from build123d import *

# Parameters (mm, degrees)
SKETCH042_R              = 1.9
PAD007_DEPTH             = 1.9
POCKET024_DEPTH          = 1.2
SKETCH044_R              = 1
PAD008_DEPTH             = 12
FILLET005_R              = 0.2
BODY008_PLACEMENT_ANGLE  = 90
CLONE004_PLACEMENT_ANGLE = 90


with BuildPart() as part:
    # Sketch042 → Pad007 (new body)
    with BuildSketch(Plane.XY):
        Circle(SKETCH042_R)
    extrude(amount=PAD007_DEPTH)

    # Sketch043 (on Face3 of Pad007) → Pocket024 (cut)
    with BuildSketch(Plane.XY.offset(1.9)):
        Polygon((0.866025, 0), (0.433013, 0.75), (-0.433013, 0.75), (-0.866025, 0), (-0.433013, -0.75), (0.433013, -0.75), align=None)
    extrude(amount=-POCKET024_DEPTH, mode=Mode.SUBTRACT)

    # Sketch044 → Pad008 (join)
    with BuildSketch(Plane.XY):
        Circle(SKETCH044_R)
    extrude(amount=-PAD008_DEPTH)

    # Fillet005
    fillet005_edges = [part.edges().sort_by_distance(p)[0] for p in [
        (-1.9, 0, 1.9),
        (-0.649519, 0.375, 1.9),
        (-0.649519, -0.375, 1.9),
        (0, -0.75, 1.9),
        (0.649519, -0.375, 1.9),
        (0.649519, 0.375, 1.9),
        (0, 0.75, 1.9),
    ]]
    fillet(fillet005_edges, radius=FILLET005_R)


with BuildPart() as part_1:
    # Body008 placement: moved
    add(part.part.moved(Location((40, -5, 15))).rotate(Axis((40, -5, 15), (1, 0, 0)), BODY008_PLACEMENT_ANGLE))


with BuildPart() as part_2:
    # Clone004 placement: moved
    add(part_1.part.moved(Location((-40, -15, -5))).rotate(Axis((-40, -15, -5), (-1, 0, 0)), CLONE004_PLACEMENT_ANGLE))


with BuildPart() as part_3:
    # Body011 placement: moved
    add(part_2.part.moved(Location((67, -5, 21))))


solid = part_3.part
The listing builds one solid part. Answer for the finished solid, in the listing's coordinates (mm). A direction names the side the tool comes from. Coordinates: 2 decimals unless noted, no trailing zeros. Loops run counter-clockwise (first coordinate to the right, second up) from the corner with the lowest first, then second, coordinate; pieces in that order, holes last. Notation, with made-up numbers: (26.5, 36.25) -> (35.5, 36.25) arc R7 ccw to (35.5, 48.25) -> close; hole circle Ø2 at (14, 86.5). An arc over 180 degrees is marked (long way). Answer in a Markdown table with one row per item. Add a question column.
1. Determine the mould class of faces 1 (the cylindrical face through (66, -5, 15)), 2 (the flat face through (68, -6, 22.9)), 3 (the flat face through (67, -5.75, 22)) for opening direction X: +X half, -X half, draft (parallel to the pull), parting line (faces both ways), or undercut.
2. Consider line 1 (Z direction, x = 68.35, y = -5.65); line 2 (X direction, y = -4.5, z = 14.5); line 3 (Z direction, x = 67.4, y = -4.4). Determine where each line is inside the solid, lowest interval first. Write a range as [from, to].
3. A flat-ended cylindrical pin translates along its axis: P1, Ø2, axis at y = -5.5, z = 15.5, coming from the +X side. Find the tip coordinate at first contact, or state that the pin passes through.
4. The part is cut by section A-A, the plane x = 67. Write down the section's boundary in (y, z).
5. The part is cut by section B-B, the plane z = 14.75. Write down the section's boundary in (x, y), then the cut area to 3 significant figures.
6. For faces 4 (the flat face through (67, -5, 21.7)), 5 (the flat face through (68, -6, 21)), 6 (the flat face through (67, -5, 9)), determine the directions among +Z, -Z, +X, -X, +Y, -Y from which every point of the face is accessible in a straight line to the end or side of a thin tool.
Answer below:
| question | item | result |
|---|---|---|
| 1 | face 1 | parting line |
| 1 | face 2 | draft |
| 1 | face 3 | undercut |
| 2 | line 1 | [21, 22.9] |
| 2 | line 2 | [66.13, 67.87] |
| 2 | line 3 | [9, 21.7] |
| 3 | P1 | x = 68 |
| 4 | outline | (-6.9, 21) -> (-6, 21) -> (-6, 9) -> (-4, 9) -> (-4, 21) -> (-3.1, 21) -> (-3.1, 22.7) arc R0.2 ccw to (-3.3, 22.9) -> (-4.05, 22.9) arc R0.2 ccw to (-4.25, 22.7) -> (-4.25, 21.7) -> (-5.75, 21.7) -> (-5.75, 22.7) arc R0.2 ccw to (-5.95, 22.9) -> (-6.7, 22.9) arc R0.2 ccw to (-6.9, 22.7) -> close |
| 5 | outline | circle Ø2 at (67, -5) |
| 5 | area | 3.14 mm2 |
| 6 | face 4 | +Z |
| 6 | face 5 | -Z |
| 6 | face 6 | -Z, +X, -X, +Y, -Y |
